Answer from the drawing. Dimensions are ordinates in mm from the lowest x, y and z of the part. A direction names the side the tool comes from. Give positions to 0.01 mm unless a question says otherwise; leave off trailing zeros. Write each loop counter-clockwise with the first axis right and the second up, starting at its lowest first coordinate (ties: lowest second). Pieces come first, ordered by that corner, then holes.
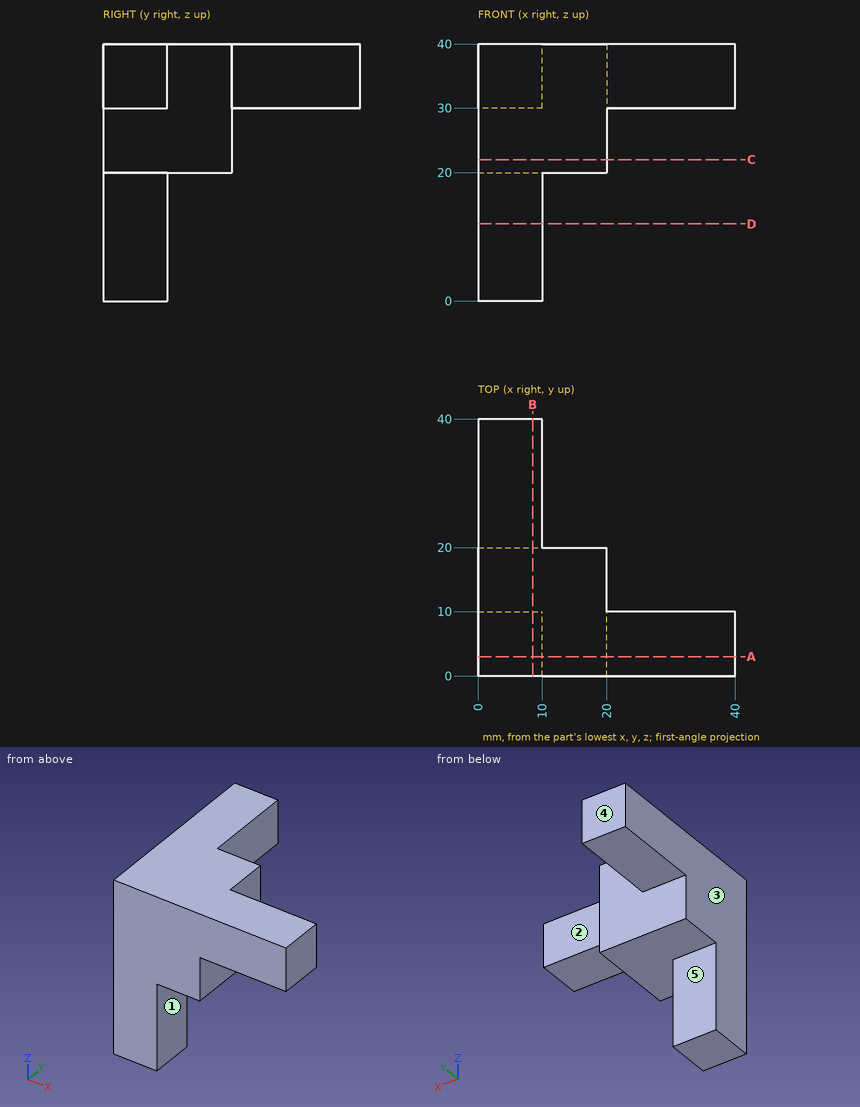
Item 1: Consider probe 1 along Y at (x, z) = (8.5, 4.5); probe 2 along X at (y, z) = (19, 38); probe 3 along Z at (x, y) = (14, 12). Determine where each line is inside the solid, lowest interval first.
Conclusion:
probe 1: y = 0 to 10
probe 2: x = 0 to 20
probe 3: z = 20 to 40
Item 2: Which of the six approach directions +Z, -Z, +X, -X, +Y, -Y give full straight-line access (tool end or side, diameter ignored) to the marked faces 1, 2, 3, 4 and 5?
Conclusion:
face 1: -Z, +X, +Y, -Y
face 2: +Z, -Z, +X, +Y
face 3: +Z, -Z, -X, +Y, -Y
face 4: +Z, -Z, +X, -X, +Y
face 5: -Z, +X, -X, +Y
Item 3: A cutting plane is placed at D-D, the plane z = 12. Give the vertices of the cut face in (x, y), plus the area to 3 significant figures.
Conclusion:
outline: (0, 0) - (10, 0) - (10, 10) - (0, 10) - close
area: 100 mm2
Item 4: A cutting plane is placed at A-A, the plane y = 3. Give the vertices of the cut face in (x, z), plus the area to 3 significant figures.
Conclusion:
outline: (0, 0) - (10, 0) - (10, 20) - (20, 20) - (20, 30) - (40, 30) - (40, 40) - (0, 40) - close
area: 800 mm2
Item 5: A cutting plane is placed at C-C, the plane z = 22. Give the vertices of the cut face in (x, y).
Conclusion:
outline: (0, 0) - (20, 0) - (20, 20) - (0, 20) - close
Item 6: Each of these flat-tipped pins is pushed along its axis until it touches: P1, Ø11, axis at x = 7.5, z = 5.5, coming from the +Y side; P2, Ø12, axis at x = 26.5, z = 10, coming from the +Y side; P3, Ø2, axis at x = 19.5, z = 32.5, coming from the +Y side; P4, Ø6, axis at x = 13.5, y = 12.5, coming from the -Z side. Where does it stop, or does it pass through?
Conclusion:
P1: stops at y = 10
P2: passes through
P3: stops at y = 20
P4: stops at z = 20
